```python
from build123d import *

# Parameters (mm, degrees)
SKETCH1_W           = 74
SKETCH1_H           = 74
BOSS_EXTRUDE1_DEPTH = 2
SKETCH2_W           = 60
SKETCH2_H           = 74
BOSS_EXTRUDE2_DEPTH = 30
SKETCH3_R           = 2
CUT_EXTRUDE1_DEPTH  = 2


with BuildPart() as part:
    # Sketch1 → Boss-Extrude1 (new body)
    with BuildSketch(Plane(origin=(0, 0, 0), x_dir=(1, 0, 0), z_dir=(0, 1, 0))):
        with Locations((37, 37)):
            Rectangle(SKETCH1_W, SKETCH1_H)
    extrude(amount=BOSS_EXTRUDE1_DEPTH)

    # Sketch2 → Boss-Extrude2 (add)
    with BuildSketch(Plane(origin=(0, 2, 0), x_dir=(1, 0, 0), z_dir=(0, 1, 0))):
        with Locations((37, 37)):
            Rectangle(SKETCH2_W, SKETCH2_H)
    extrude(amount=BOSS_EXTRUDE2_DEPTH)

    # Sketch3 → Cut-Extrude1 (cut)
    with BuildSketch(Plane.XZ):
        with Locations(Location((4.5, -37, 0), (0, 0, 270))):
            Circle(SKETCH3_R)
        with Locations(Location((69.5, -37, 0), (0, 0, 90))):
            Circle(SKETCH3_R)
    extrude(amount=-CUT_EXTRUDE1_DEPTH, mode=Mode.SUBTRACT)


solid = part.part
```
Input: part model. Units: mm. Frame: model coordinates. A direction names the side the tool comes from. Give positions to 0.01 mm unless a question says otherwise; leave off trailing zeros. Order: outer loops, then holes, each group sorted by start corner. A loop starts at its lowest first (then second) coordinate and runs counter-clockwise, first axis right, second up. Notation, with made-up numbers: M 61.5,-36.5 L 109.5,-36.5 A27 cw 109.5,2.5 Z; hole C -28,15.5 d9. An arc over 180 degrees is marked long. One line per question, with ' | ' between items. Start each with the question number.
1. Material intervals for probe 1 along X at (y, z) = (1, -37); probe 2 along Z at (x, y) = (69.5, 0.7); probe 3 along Y at (x, z) = (5.5, -4), sorted ascending. Write a range as [from, to].
2. Access query for faces 4 (the face through (36, 16, 0)), 5 (the face through (67, 17, -36)), 6 (the face through (2, 2, -38)). Directions: +Z, -Z, +X, -X, +Y, -Y. A direction counts if a zero-diameter tool reaches every point of the face in a straight line with its end or side. Return the directions, or none.
3. Section query D-D (y = 10.5). Return the cut outline in (x, z).
4. First-contact query: pin 1 Ø2 at (x, z) = (3.5, -34.5) entering from +Y; pin 2 Ø9 at (y, z) = (14.5, -32) entering from +X; pin 3 Ø6.5 at (x, z) = (69.5, -37) entering from +Y. Flat tips, straight axial feed; report the tip coordinate or a pass-through.
5. Pull-direction query (X, two-part tool) for faces 1 (the face through (67.517, 0.986, -37.26)), 2 (the face through (36, 16, -74)), 3 (the face through (0, 1, -36)); classes: released by +X, released by -X, zero draft, split by the parting line, or undercut.
6. Section query C-C (z = -4.5). Return the cut outline in (x, y).
7. Section query A-A (z = -37). Return the cut outline in (x, y).
8. Section query B-B (x = 69.5). Return the cut outline in (y, z).
Here are the results:
1) probe 1: [0, 2.5], [6.5, 67.5], [71.5, 74] | probe 2: [-74, -39], [-35, 0] | probe 3: [0, 2]
2) face 4: +Z, +X, -X, +Y, -Y | face 5: +Z, -Z, +X, +Y | face 6: +Z, -Z, -X, +Y
3) outline: M 7,-74 L 67,-74 L 67,0 L 7,0 Z
4) pin 1: y = 2 | pin 2: x = 67 | pin 3: y = 32
5) face 1: undercut | face 2: zero draft | face 3: released by -X
6) outline: M 0,0 L 74,0 L 74,2 L 67,2 L 67,32 L 7,32 L 7,2 L 0,2 Z
7) outline: M 0,0 L 2.5,0 L 2.5,2 L 0,2 Z; M 6.5,0 L 67.5,0 L 67.5,2 L 67,2 L 67,32 L 7,32 L 7,2 L 6.5,2 Z; M 71.5,0 L 74,0 L 74,2 L 71.5,2 Z
8) outline: M 0,-74 L 2,-74 L 2,-39 L 0,-39 Z; M 0,-35 L 2,-35 L 2,0 L 0,0 Z
